```python
from build123d import *

# Parameters (mm, degrees)
ESQUISSE2_R                  = 109
BOSS_EXTRU_1_DEPTH           = 3
ESQUISSE3_W                  = 58
ESQUISSE3_H                  = 42.41769301
ENL_V_MAT_EXTRU_1_DEPTH      = 3
D_GAGEMENT_M31_D             = 3.4
D_GAGEMENT_M31_CSINK_D       = 3.45
D_GAGEMENT_M31_CSINK_ANGLE   = 90
R_P_TITION_CIRCULAIRE1_COUNT = 3


with BuildPart() as part:
    # Esquisse2 → Boss.-Extru.1 (new body)
    with BuildSketch(Plane.XY):
        Circle(ESQUISSE2_R)
    extrude(amount=BOSS_EXTRU_1_DEPTH)

    # Esquisse3 → Enlèv. mat.-Extru.1 (cut)
    with BuildSketch(Plane.XY.offset(3)):
        with Locations((0, -99.780250798)):
            Rectangle(ESQUISSE3_W, ESQUISSE3_H)
        Polygon((-90.279631846, 85.609285361), (-119.279631846, 35.379811942), (-82.544832128, 14.170965437), (-53.544832128, 64.400438856), align=None)
        Polygon((119.279631846, 35.379811942), (90.279631846, 85.609285361), (53.544832128, 64.400438856), (82.544832128, 14.170965437), align=None)
    extrude(amount=-ENL_V_MAT_EXTRU_1_DEPTH, mode=Mode.SUBTRACT)

    # Dégagement M31 (through all)
    with Locations(Plane.XY.offset(3)):
        with Locations((-48.088245044, -79.426901276), (48.068989794, -79.426901276)):
            d_gagement_m31 = CounterSinkHole(D_GAGEMENT_M31_D / 2, D_GAGEMENT_M31_CSINK_D / 2, counter_sink_angle=D_GAGEMENT_M31_CSINK_ANGLE)

    # Répétition circulaire1: Dégagement M31 ×3 about axis
    r_p_tition_circulaire1_axis = Axis((5.584e-06, 0.046063312, 0), (0, 0, 1))
    for i in range(1, R_P_TITION_CIRCULAIRE1_COUNT):
        add(d_gagement_m31.rotate(r_p_tition_circulaire1_axis, i * 360 / R_P_TITION_CIRCULAIRE1_COUNT), mode=Mode.SUBTRACT)


solid = part.part
```
The model under review builds one solid part; all positions refer to its coordinate system, in mm. A direction names the side the tool comes from. Round coordinates to 2 decimals unless told otherwise and drop trailing zeros. Loops run counter-clockwise (first coordinate to the right, second up) from the corner with the lowest first, then second, coordinate; pieces in that order, holes last.
Item 1: Take a section at C-C (z = 1). Write out the cut boundary in (x, y), then the cut area to 3 significant figures.
Determined:
outline: (-105.49, 27.42) arc R109 ccw to (-29, -105.07) - (-29, -78.57) - (29, -78.57) - (29, -105.07) arc R109 ccw to (105.49, 27.42) - (82.54, 14.17) - (53.54, 64.4) - (76.49, 77.65) arc R109 ccw to (-76.49, 77.65) - (-53.54, 64.4) - (-82.54, 14.17) - close; hole circle Ø3.4 at (-92.86, -1.85); hole circle Ø3.4 at (-48.09, -79.43); hole circle Ø3.4 at (-44.78, 81.43); hole circle Ø3.4 at (44.79, 81.41); hole circle Ø3.4 at (48.07, -79.43); hole circle Ø3.4 at (92.87, -1.86)
area: 32,200 mm2
Item 2: Take a section at A-A (x = 74). Write out the cut boundary in (y, z), then the cut area to 3 significant figures.
Determined:
outline: (-80.03, 0) - (28.97, 0) - (28.97, 3) - (-80.03, 3) - close; (76.21, 0) - (80.03, 0) - (80.03, 3) - (76.21, 3) - close
area: 338 mm2
Item 3: Take a section at B-B (y = 91). Write out the cut boundary in (x, z).
Determined:
outline: (-60, 0) - (60, 0) - (60, 3) - (-60, 3) - close
Item 4: Take a section at D-D (x = 7.5). Write out the cut boundary in (y, z), then the cut area to 3 significant figures.
Determined:
outline: (-78.57, 0) - (108.74, 0) - (108.74, 3) - (-78.57, 3) - close
area: 562 mm2
Item 5: Clearance check with flat-ended pins moving along their axes: pin 1 Ø1.5 at (x, y) = (27, -46) entering from -Z; pin 2 Ø1.5 at (y, z) = (54, 0.5) entering from +X; pin 3 Ø1.5 at (y, z) = (20, 2) entering from +X; pin 4 Ø2 at (x, y) = (48.07, -79.43) entering from -Z. State where each tip first meets the part, or that it passes through.
Determined:
pin 1: stops at z = 0
pin 2: stops at x = 59.98
pin 3: stops at x = 107.29
pin 4: passes through
Item 6: Mouldability with a two-part tool opening along X and no side actions: class faces 1 (the face through (-94.985, -53.469, 1.479)), 2 (the face through (-2, 3, 0)), 3 (the face through (-68.25, 38.93, 1.52)) as released by +X, released by -X, zero draft, split by the parting line, or undercut.
Determined:
face 1: released by -X
face 2: zero draft
face 3: undercut
Item 7: For line 1 (X direction, y = 15, z = 0.4); line 2 (X direction, y = 3, z = 0.45); line 3 (Y direction, x = 63, z = 2.45), list the stretches that pass through material, from the lowest coordinate up.
Determined:
line 1: x = -107.96 to -83.98, -82.07 to 82.07, 83.98 to 107.96
line 2: x = -108.96 to 108.96
line 3: y = -88.95 to 48.02, 69.86 to 88.95
Item 8: For faces 4 (the face through (-64.859, 70.933, 1.521)), 5 (the face through (65.18, 71.12, 1.52)), 6 (the face through (-94.2, 20.9, 1.5)), 7 (the face through (-2, 3, 3)), 8 (the face through (67.84, 39.64, 1.52)), list the 3-axis set-ups (+Z, -Z, +X, -X, +Y, -Y) from which the entire face can be reached by the end or side of a thin tool; tool diameter is ignored.
Determined:
face 4: +Z, -Z, -X
face 5: +Z, -Z, +X
face 6: +Z, -Z, +Y
face 7: +Z, +X, -X, +Y, -Y
face 8: +Z, -Z
